Build history of the part. All positions in model axes, mm. Face numbers are marked on the shaded views. Round coordinates to 2 decimals unless told otherwise and drop trailing zeros. Write each loop counter-clockwise with the first axis right and the second up, starting at its lowest first coordinate (ties: lowest second). Pieces come first, ordered by that corner, then holes. Notation, with made-up numbers: (36.5, 31.25) -> (62.5, 31.25) arc R20 cw to (62.5, 37.25) -> close; hole circle Ø11 at (84, 17.5). An arc over 180 degrees is marked (long way). Return JSON: item names as keys, results as strings.
from build123d import *

# Parameters (mm, degrees)
SKETCH1_W           = 266.7
SKETCH1_H           = 304.8
BOSS_EXTRUDE1_DEPTH = 25.4
SKETCH2_W           = 260.35
SKETCH2_H           = 22.225
CUT_EXTRUDE1_DEPTH  = 12700
CUT_EXTRUDE2_DEPTH  = 12700
CUT_EXTRUDE10_DEPTH = 12700
SKETCH5_R           = 2.38125
CUT_EXTRUDE11_DEPTH = 267.7
SKETCH6_R           = 2.38125
CUT_EXTRUDE12_DEPTH = 4.175
SKETCH7_R           = 14.2875
CUT_EXTRUDE13_DEPTH = 3.175
SKETCH8_R           = 2.38125
CUT_EXTRUDE14_DEPTH = 4.175
CUT_EXTRUDE15_DEPTH = 267.7


with BuildPart() as part:
    # Sketch1 → Boss-Extrude1 (new body)
    with BuildSketch(Plane(origin=(0, 0, 0), x_dir=(1, 0, 0), z_dir=(0, 1, 0))):
        with Locations((46.828595318, 35.997491639)):
            Rectangle(SKETCH1_W, SKETCH1_H)
    extrude(amount=BOSS_EXTRUDE1_DEPTH)

    # Sketch2 → Cut-Extrude1 (cut)
    with BuildSketch(Plane.XY.offset(116.402508361)):
        with Locations((46.828595318, 14.2875)):
            Rectangle(SKETCH2_W, SKETCH2_H)
    extrude(amount=-CUT_EXTRUDE1_DEPTH, mode=Mode.SUBTRACT)

    # Sketch3 → Cut-Extrude2 (cut)
    with BuildSketch(Plane(origin=(0, 3.175, 0), x_dir=(1, 0, 0), z_dir=(0, 1, 0))):
        with BuildLine():
            ThreePointArc((65.878595318, -91.002508361), (61.388467257, -89.142636422), (59.528595318, -84.652508361))
            Line((59.528595318, -84.652508361), (59.528595318, 16.947491639))
            ThreePointArc((59.528595318, 16.947491639), (61.388467257, 21.437619699), (65.878595318, 23.297491639))
            Line((65.878595318, 23.297491639), (145.253595318, 23.297491639))
            ThreePointArc((145.253595318, 23.297491639), (149.743723378, 21.437619699), (151.603595318, 16.947491639))
            Line((151.603595318, 16.947491639), (151.603595318, -84.652508361))
            ThreePointArc((151.603595318, -84.652508361), (149.743723378, -89.142636422), (145.253595318, -91.002508361))
            Line((145.253595318, -91.002508361), (65.878595318, -91.002508361))
        make_face()
        with BuildLine():
            ThreePointArc((145.253595318, 162.997491639), (149.743723378, 161.137619699), (151.603595318, 156.647491639))
            Line((151.603595318, 156.647491639), (151.603595318, 55.047491639))
            ThreePointArc((151.603595318, 55.047491639), (149.743723378, 50.557363578), (145.253595318, 48.697491639))
            Line((145.253595318, 48.697491639), (65.878595318, 48.697491639))
            ThreePointArc((65.878595318, 48.697491639), (61.388467257, 50.557363578), (59.528595318, 55.047491639))
            Line((59.528595318, 55.047491639), (59.528595318, 156.647491639))
            ThreePointArc((59.528595318, 156.647491639), (61.388467257, 161.137619699), (65.878595318, 162.997491639))
            Line((65.878595318, 162.997491639), (145.253595318, 162.997491639))
        make_face()
        with BuildLine():
            ThreePointArc((27.778595318, 162.997491639), (32.268723378, 161.137619699), (34.128595318, 156.647491639))
            Line((34.128595318, 156.647491639), (34.128595318, 55.047491639))
            ThreePointArc((34.128595318, 55.047491639), (32.268723378, 50.557363578), (27.778595318, 48.697491639))
            Line((27.778595318, 48.697491639), (-51.596404682, 48.697491639))
            ThreePointArc((-51.596404682, 48.697491639), (-56.086532743, 50.557363578), (-57.946404682, 55.047491639))
            Line((-57.946404682, 55.047491639), (-57.946404682, 156.647491639))
            ThreePointArc((-57.946404682, 156.647491639), (-56.086532743, 161.137619699), (-51.596404682, 162.997491639))
            Line((-51.596404682, 162.997491639), (27.778595318, 162.997491639))
        make_face()
        with BuildLine():
            Line((-57.946404682, -84.652508361), (-57.946404682, 16.947491639))
            ThreePointArc((-57.946404682, 16.947491639), (-56.086532743, 21.437619699), (-51.596404682, 23.297491639))
            Line((-51.596404682, 23.297491639), (27.778595318, 23.297491639))
            ThreePointArc((27.778595318, 23.297491639), (32.268723378, 21.437619699), (34.128595318, 16.947491639))
            Line((34.128595318, 16.947491639), (34.128595318, -84.652508361))
            ThreePointArc((34.128595318, -84.652508361), (32.268723378, -89.142636422), (27.778595318, -91.002508361))
            Line((27.778595318, -91.002508361), (-51.596404682, -91.002508361))
            ThreePointArc((-51.596404682, -91.002508361), (-56.086532743, -89.142636422), (-57.946404682, -84.652508361))
        make_face()
    extrude(amount=-CUT_EXTRUDE2_DEPTH, mode=Mode.SUBTRACT)

    # Sketch4 → Cut-Extrude10 (cut)
    with BuildSketch(Plane(origin=(180.178595318, 0, 0), x_dir=(0, 0, -1), z_dir=(1, 0, 0))):
        Polygon((162.997491639, 25.4), (188.397491639, 0), (188.397491639, 25.4), align=None)
        Polygon((-116.402508361, 0), (-91.002508361, 25.4), (-116.402508361, 25.4), align=None)
    extrude(amount=-CUT_EXTRUDE10_DEPTH, mode=Mode.SUBTRACT)

    # Sketch5 → Cut-Extrude11 (cut, through all)
    with BuildSketch(Plane(origin=(180.178595318, 0, 0), x_dir=(0, 0, -1), z_dir=(1, 0, 0))):
        with Locations((86.797491639, 12.7)):
            Circle(SKETCH5_R)
        with Locations((35.997491639, 12.7)):
            Circle(SKETCH5_R)
        with Locations((61.397491639, 12.7)):
            Circle(SKETCH5_R)
        with Locations((10.597491639, 12.7)):
            Circle(SKETCH5_R)
        with Locations((-14.802508361, 12.7)):
            Circle(SKETCH5_R)
    extrude(amount=-CUT_EXTRUDE11_DEPTH, mode=Mode.SUBTRACT)

    # Sketch6 → Cut-Extrude12 (cut, through all)
    with BuildSketch(Plane(origin=(0, 3.175, 0), x_dir=(1, 0, 0), z_dir=(0, 1, 0))):
        with Locations((46.828595318, 175.697491639)):
            Circle(SKETCH6_R)
        with Locations((21.428595318, 175.697491639)):
            Circle(SKETCH6_R)
        with Locations((-3.971404682, 175.697491639)):
            Circle(SKETCH6_R)
        with Locations((72.228595318, 175.697491639)):
            Circle(SKETCH6_R)
        with Locations((97.628595318, 175.697491639)):
            Circle(SKETCH6_R)
    extrude(amount=-CUT_EXTRUDE12_DEPTH, mode=Mode.SUBTRACT)

    # Sketch7 → Cut-Extrude13 (cut)
    with BuildSketch(Plane(origin=(0, 3.175, 0), x_dir=(1, 0, 0), z_dir=(0, 1, 0))):
        with Locations((-68.106404682, -97.987508361)):
            Circle(SKETCH7_R)
        with Locations((161.763595318, -97.987508361)):
            Circle(SKETCH7_R)
    extrude(amount=-CUT_EXTRUDE13_DEPTH, mode=Mode.SUBTRACT)

    # Sketch8 → Cut-Extrude14 (cut, through all)
    with BuildSketch(Plane(origin=(0, 3.175, 0), x_dir=(1, 0, 0), z_dir=(0, 1, 0))):
        with Locations((167.478595318, 35.997491639)):
            Circle(SKETCH8_R)
        with Locations((167.478595318, 61.397491639)):
            Circle(SKETCH8_R)
        with Locations((167.478595318, 86.797491639)):
            Circle(SKETCH8_R)
        with Locations((167.478595318, 10.597491639)):
            Circle(SKETCH8_R)
        with Locations((167.478595318, -14.802508361)):
            Circle(SKETCH8_R)
        with Locations((-73.821404682, -14.802508361)):
            Circle(SKETCH8_R)
        with Locations((-73.821404682, 10.597491639)):
            Circle(SKETCH8_R)
        with Locations((-73.821404682, 35.997491639)):
            Circle(SKETCH8_R)
        with Locations((-73.821404682, 61.397491639)):
            Circle(SKETCH8_R)
        with Locations((-73.821404682, 86.797491639)):
            Circle(SKETCH8_R)
    extrude(amount=-CUT_EXTRUDE14_DEPTH, mode=Mode.SUBTRACT)

    # Sketch9 → Cut-Extrude15 (cut, through all)
    with BuildSketch(Plane.ZY.offset(86.521404682)):
        Polygon((-175.697491639, 20.032348419), (-182.047491639, 16.366174209), (-182.047491639, 9.033825791), (-175.697491639, 5.367651581), (-169.347491639, 9.033825791), (-169.347491639, 16.366174209), align=None)
    extrude(amount=-CUT_EXTRUDE15_DEPTH, mode=Mode.SUBTRACT)


solid = part.part
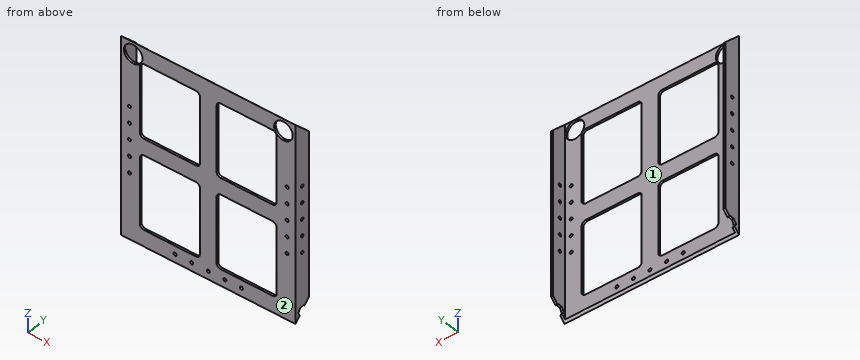
Q1. Saw through at B-B on x = 104. List the corners of the cut face in (y, z) (1 decimal).
Verdict:
{"outline": "(0, -188.4) -> (3.2, -185.2) -> (3.2, -163) -> (0, -163) -> close; (0, -48.7) -> (3.2, -48.7) -> (3.2, -23.3) -> (0, -23.3) -> close; (0, 91) -> (3.2, 91) -> (3.2, 113.2) -> (0, 116.4) -> close"}
Q2. Pin check, flat tips, straight feed: pin 1 Ø2.5 at (x, y) = (103.5, 1) entering from +Z; pin 2 Ø2.5 at (x, y) = (-15.5, 2.5) entering from +Z; pin 3 Ø7.5 at (x, z) = (46.83, -175.7) entering from +Y (3 decimals). Stop position of each tip, or through.
Verdict:
{"pin 1": "stops at z = 116.4", "pin 2": "stops at z = 115.15", "pin 3": "stops at y = 3.175"}
Q3. Saw through at A-A on z = -138. List the corners of the cut face in (x, y) (3 decimals), then the cut area to 3 significant figures.
Verdict:
{"outline": "(-86.521, 0) -> (-57.946, 0) -> (-57.946, 3.175) -> (-83.346, 3.175) -> (-83.346, 25.4) -> (-86.521, 25.4) -> close; (34.129, 0) -> (59.529, 0) -> (59.529, 3.175) -> (34.129, 3.175) -> close; (151.604, 0) -> (180.179, 0) -> (180.179, 25.4) -> (177.004, 25.4) -> (177.004, 3.175) -> (151.604, 3.175) -> close", "area": "403 mm²"}
Q4. Two-plate mould, pull along X, no slides. Class the marked faces 1 and 2: +X half, -X half, draft (parallel to the pull), parting line (faces both ways), or undercut.
Verdict:
{"face 1": "undercut", "face 2": "draft"}
Q5. Wall check: L1, parallel to X at y = 2, z = 48; L2, parallel to X at y = 6.5, z = -4; L3, parallel to Z at x = -33, y = 2. Give the ranges that are in metal, low to high.
Verdict:
{"L1": "x = -86.52 to -57.95, 34.13 to 59.53, 151.6 to 180.18", "L2": "x = -86.52 to -83.35, 177 to 180.18", "L3": "z = -186.4 to -163, -48.7 to -23.3, 91 to 114.4"}
